Here's how the part is built. I have some questions about the finished solid (model axes, mm). A direction names the side the tool comes from. Give positions to 0.01 mm unless a question says otherwise; leave off trailing zeros. Loops run counter-clockwise (first coordinate to the right, second up) from the corner with the lowest first, then second, coordinate; pieces in that order, holes last. Notation, with made-up numbers: (44.25, 22.5) -> (61.25, 22.5) arc R34 cw to (61.25, 60.5) -> close; hole circle Ø10 at (26, 46.25). An arc over 180 degrees is marked (long way). Answer in a Markdown table with one row per item. Add a question column.
Item 1: If I drill on line 1 (X direction, y = 13, z = 66.5); line 2 (Y direction, x = -5, z = 61); line 3 (X direction, y = -24, z = 64.75), over which ranges is the centre line in solid material (lowest first)?
Item 2: If we section it at A-A (y = 0): Write out the boundary of the cut face in (x, z) (3 decimals), then the cut area to 3 significant figures.
Item 3: We'd pull the mould along Y, two halves only. Please class faces 6 (the face through (0, 13.5, 46)), 7 (the face through (0, -16, 55)), 8 (the face through (-1.172, 8.923, 53.591)), 9 (the face through (0, -13.5, 56)): released by +Y, released by -Y, zero draft, split by the parting line, or undercut.
Item 4: Which directions (+Z, -Z, +X, -X, +Y, -Y) give clear straight access to the entire face, cutting with the end or side of a thin tool? Please do faces 1 (the face through (0, 10, 65)), 2 (the face through (-14.2, 10.1, 63)), 3 (the face through (0, -13.5, 46)), 4 (the face through (0, -18.5, 51)), 5 (the face through (8.73, 6.69, 45.67)).
Item 5: If we section it at D-D (y = -6): Write out the boundary of the cut face in (x, z).
Item 6: For P1, Ø5, axis at x = 9.5, z = 47.5, coming from the -Y side; P2, Ø12, axis at x = 13, z = 58, coming from the +Y side; P3, Ø5, axis at x = -1.5, y = -3, coming from the -Z side; P4, Ø1, axis at y = 1, z = 47, coming from the +X side, each with a flat end and sliding along its axis, tell me the tip position at first contact or that it passes through.
Item 7: If we section it at C-C (y = -24): Write out the boundary of the cut face in (x, z), then the cut area to 3 significant figures.
```python
from build123d import *

# Parameters (mm, degrees)
BOSS_EXTRUDE1_DEPTH      = 13.5
BOSS_EXTRUDE2_DEPTH      = 18.5
BOSS_EXTRUDE3_DEPTH      = 5
SKETCH4_W                = 45.922011884
SKETCH4_H                = 20
BOSS_EXTRUDE4_DEPTH      = 13.5
SKETCH2_R                = 4
CUT_EXTRUDE1_DEPTH       = 268.629329099
SKETCH5_R                = 8
CUT_EXTRUDE2_DEPTH       = 4
SKETCH6_R                = 9
CUT_EXTRUDE3_DEPTH       = 12
SKETCH7_R                = 12.5
CUT_EXTRUDE4_DEPTH       = 5
BOSS_EXTRUDE5_DEPTH      = 13.5
CUT_EXTRUDE5_REACH       = 210.1
CUT_EXTRUDE5_END_RADIUS  = 45
SKETCH8_R                = 9
CUT_EXTRUDE6_REACH       = 210.1
SKETCH10_R               = 4.5
SKETCH18_R               = 11
CUT_EXTRUDE9_DEPTH       = 47
CUT_EXTRUDE10_DEPTH      = 268.629329099
CUT_EXTRUDE10_DEPTH_BACK = 268.629329099
SKETCH19_W               = 45.922011884
SKETCH19_H               = 198
SKETCH30_R               = 8.025
CUT_EXTRUDE13_DEPTH      = 4
BOSS_EXTRUDE9_DEPTH      = 16
M5_TAPPED_HOLE2_D        = 4.2
CUT_EXTRUDE17_DEPTH      = 3
M2_TAPPED_HOLE1_D        = 1.6
M2_TAPPED_HOLE1_DEPTH    = 8
M2_TAPPED_HOLE1_TIP      = 0.480688495


with BuildPart() as part:
    # Sketch1 → Boss-Extrude1 (new, symmetric)
    with BuildSketch(Plane(origin=(0, 0, 0), x_dir=(1, 0, 0), z_dir=(0, 1, 0))):
        with BuildLine():
            ThreePointArc((17.220754456, -41.574578963), (0, -45), (-17.220754456, -41.574578963))
            Line((-17.220754456, -41.574578963), (-22.961005942, -55.432771951))
            ThreePointArc((-22.961005942, -55.432771951), (0, -60), (22.961005942, -55.432771951))
            Line((22.961005942, -55.432771951), (17.220754456, -41.574578963))
        make_face()
    extrude(amount=BOSS_EXTRUDE1_DEPTH, both=True)

    # Sketch1_3 → Boss-Extrude2 (add, symmetric)
    with BuildSketch(Plane(origin=(0, 0, 0), x_dir=(1, 0, 0), z_dir=(0, 1, 0))):
        with BuildLine():
            ThreePointArc((19.134171618, -46.193976626), (0, -50), (-19.134171618, -46.193976626))
            Line((-19.134171618, -46.193976626), (-21.04758878, -50.813374288))
            ThreePointArc((-21.04758878, -50.813374288), (0, -55), (21.04758878, -50.813374288))
            Line((21.04758878, -50.813374288), (19.134171618, -46.193976626))
        make_face()
    extrude(amount=BOSS_EXTRUDE2_DEPTH, both=True)

    # Sketch3 → Boss-Extrude3 (add, symmetric)
    with BuildSketch(Plane.XZ):
        with BuildLine():
            Line((-22.961005942, 266), (-22.961005942, 55.432771951))
            ThreePointArc((-22.961005942, 55.432771951), (-20.481139434, 56.39612511), (-17.961005942, 57.248600555))
            Line((-17.961005942, 57.248600555), (-17.961005942, 246))
            Line((-17.961005942, 246), (17.961005942, 246))
            Line((17.961005942, 246), (17.961005942, 57.248600555))
            ThreePointArc((17.961005942, 57.248600555), (20.481139434, 56.39612511), (22.961005942, 55.432771951))
            Line((22.961005942, 55.432771951), (22.961005942, 266))
            Line((22.961005942, 266), (-22.961005942, 266))
        make_face()
    extrude(amount=BOSS_EXTRUDE3_DEPTH, both=True)

    # Sketch4 → Boss-Extrude4 (add, symmetric)
    with BuildSketch(Plane(origin=(0, 0, 0), x_dir=(1, 0, 0), z_dir=(0, 1, 0))):
        with Locations((0, -256)):
            Rectangle(SKETCH4_W, SKETCH4_H)
    extrude(amount=BOSS_EXTRUDE4_DEPTH, both=True)

    # Sketch2 → Cut-Extrude1 (cut, through all)
    with BuildSketch(Plane.XY):
        with Locations(Location((0, 0, 0), (0, 0, 180))):
            Circle(SKETCH2_R)
    extrude(amount=CUT_EXTRUDE1_DEPTH, mode=Mode.SUBTRACT)

    # Sketch5 → Cut-Extrude2 (cut)
    with BuildSketch(Plane(origin=(0, 0, 246), x_dir=(-1, 0, 0), z_dir=(0, 0, -1))):
        Circle(SKETCH5_R)
    extrude(amount=-CUT_EXTRUDE2_DEPTH, mode=Mode.SUBTRACT)

    # Sketch6 → Cut-Extrude3 (cut)
    with BuildSketch(Plane.XY.offset(266)):
        Circle(SKETCH6_R)
    extrude(amount=-CUT_EXTRUDE3_DEPTH, mode=Mode.SUBTRACT)

    # Sketch7 → Cut-Extrude4 (cut)
    with BuildSketch(Plane.XY.offset(266)):
        Circle(SKETCH7_R)
    extrude(amount=-CUT_EXTRUDE4_DEPTH, mode=Mode.SUBTRACT)

    # Sketch9 → Boss-Extrude5 (add, symmetric)
    with BuildSketch(Plane(origin=(0, 0, 0), x_dir=(1, 0, 0), z_dir=(0, 1, 0))):
        with BuildLine():
            Line((-22.961005942, -55.432771951), (-22.961005942, -68))
            Line((-22.961005942, -68), (22.961005942, -68))
            Line((22.961005942, -68), (22.961005942, -55.432771951))
            ThreePointArc((22.961005942, -55.432771951), (0, -60), (-22.961005942, -55.432771951))
        make_face()
    extrude(amount=BOSS_EXTRUDE5_DEPTH, both=True)

    # Cut-Extrude5: up to this cylinder (the profile starts outside it)
    cut_extrude5_end = Plane(origin=(0, 0, 0), z_dir=(0, -1, 0)) * Cylinder(CUT_EXTRUDE5_END_RADIUS, 511.2, mode=Mode.PRIVATE)
    # Sketch8 → Cut-Extrude5 (cut, up to the surface)
    with BuildSketch(Plane.XY.offset(60), mode=Mode.PRIVATE) as cut_extrude5_sk1:
        Circle(SKETCH8_R)
    cut_extrude5_tool1 = extrude(cut_extrude5_sk1.sketch, amount=-CUT_EXTRUDE5_REACH, mode=Mode.PRIVATE) - cut_extrude5_end
    add(cut_extrude5_tool1.solids().sort_by_distance((0, 0, 60))[0], mode=Mode.SUBTRACT)

    # Sketch10 → Cut-Extrude6 (cut, up to next)
    with BuildSketch(Plane.XY.offset(60), mode=Mode.PRIVATE) as cut_extrude6_sk1:
        with Locations(Location((0, 0, 0), (0, 0, 180))):
            Circle(SKETCH10_R)
    cut_extrude6_tool1 = extrude(cut_extrude6_sk1.sketch, amount=CUT_EXTRUDE6_REACH, mode=Mode.PRIVATE) & part.part
    add(cut_extrude6_tool1.solids().sort_by_distance((0, 0, 60))[0], mode=Mode.SUBTRACT)

    # Sketch18 → Cut-Extrude9 (cut)
    with BuildSketch(Plane.XY):
        with Locations(Location((0, 0, 0), (0, 0, 180))):
            Circle(SKETCH18_R)
    extrude(amount=CUT_EXTRUDE9_DEPTH, mode=Mode.SUBTRACT)

    # Sketch19 → Cut-Extrude10 (cut, two sides: drawn at the far end of the back side and taken through both)
    with BuildSketch(Plane(origin=(0, 0, 0), x_dir=(1, 0, 0), z_dir=(0, 1, 0)).offset(-CUT_EXTRUDE10_DEPTH_BACK)):
        with Locations((0, -167)):
            Rectangle(SKETCH19_W, SKETCH19_H)
    extrude(amount=CUT_EXTRUDE10_DEPTH + CUT_EXTRUDE10_DEPTH_BACK, mode=Mode.SUBTRACT)

    # Sketch23 → M5 Tapped Hole1 (revolve, cut)
    with BuildSketch(Plane(origin=(14.26606865, 8, 68), x_dir=(0, -1, 0), z_dir=(1, 0, 0))):
        Polygon((0, 0), (0, 11.3618073), (2.1, 10.1), (2.1, 0), align=None)
    m5_tapped_hole1 = revolve(axis=Axis((14.26606865, 8, 74.35), (0, 0, -1)), mode=Mode.SUBTRACT)

    # Mirror1: M5 Tapped Hole1 across plane
    add(m5_tapped_hole1.mirror(Plane(origin=(0, 0, 0), x_dir=(0, 0, 1), z_dir=(1, 0, 0))), mode=Mode.SUBTRACT)

    # Sketch30 → Cut-Extrude13 (cut)
    with BuildSketch(Plane(origin=(0, 0, 60), x_dir=(-1, 0, 0), z_dir=(0, 0, -1))):
        Circle(SKETCH30_R)
    extrude(amount=-CUT_EXTRUDE13_DEPTH, mode=Mode.SUBTRACT)

    # Sketch37 → Boss-Extrude9 (add)
    with BuildSketch(Plane.XZ.offset(13.5)):
        with BuildLine():
            Line((-22.961005942, 68), (22.961005942, 68))
            Line((22.961005942, 68), (22.961005942, 57))
            ThreePointArc((22.961005942, 57), (0, 61.450856738), (-22.961005942, 57))
            Line((-22.961005942, 57), (-22.961005942, 68))
        make_face()
    extrude(amount=BOSS_EXTRUDE9_DEPTH)

    # M5 Tapped Hole2 (through all)
    with Locations(Plane.XY.offset(68)):
        with Locations((-14.26606865, -24), (14.26606865, -24)):
            Hole(M5_TAPPED_HOLE2_D / 2)

    # Sketch40 → Cut-Extrude17 (cut)
    with BuildSketch(Plane.XY.offset(68)):
        with BuildLine():
            Line((-7, 13.5), (-7, 8))
            ThreePointArc((-7, 8), (-6.560660172, 6.939339828), (-5.5, 6.5))
            Line((-5.5, 6.5), (5.5, 6.5))
            ThreePointArc((5.5, 6.5), (6.560660172, 6.939339828), (7, 8))
            Line((7, 8), (7, 13.5))
            Line((7, 13.5), (-7, 13.5))
        make_face()
    extrude(amount=-CUT_EXTRUDE17_DEPTH, mode=Mode.SUBTRACT)

    # M2 Tapped Hole1
    with Locations(Plane.XY.offset(65)):
        with Locations((5, 10.5), (-5, 10.5)):
            Hole(M2_TAPPED_HOLE1_D / 2, depth=M2_TAPPED_HOLE1_DEPTH)
            with Locations((0, 0, -(M2_TAPPED_HOLE1_DEPTH + M2_TAPPED_HOLE1_TIP / 2))):  # 118° drill point
                Cone(0, M2_TAPPED_HOLE1_D / 2, M2_TAPPED_HOLE1_TIP, mode=Mode.SUBTRACT)


solid = part.part
```
Recorded:
| question | item | result |
|---|---|---|
| 1 | line 1 | x = -22.96 to -7, 7 to 22.96 |
| 1 | line 2 | y = -13.5 to -6.28, 6.28 to 9.7, 11.3 to 13.5 |
| 1 | line 3 | x = -22.96 to -16.37, -12.17 to 12.17, 16.37 to 22.96 |
| 2 | outline | (-22.961, 55.433) -> (-17.221, 41.575) arc R45 cw to (-11, 43.635) -> (-11, 47) -> (-9, 47) -> (-9, 60) -> (-8.025, 60) -> (-8.025, 64) -> (-4.5, 64) -> (-4.5, 68) -> (-22.961, 68) -> close; (4.5, 64) -> (8.025, 64) -> (8.025, 60) -> (9, 60) -> (9, 47) -> (11, 47) -> (11, 43.635) arc R45 cw to (17.221, 41.575) -> (22.961, 55.433) -> (22.961, 68) -> (4.5, 68) -> close |
| 2 | area | 667 mm^2 |
| 3 | face 6 | released by +Y |
| 3 | face 7 | zero draft |
| 3 | face 8 | undercut |
| 3 | face 9 | released by -Y |
| 4 | face 1 | +Z, +Y |
| 4 | face 2 | +Z |
| 4 | face 3 | -Z, -Y |
| 4 | face 4 | -Z, +X, -X, -Y |
| 4 | face 5 | -Z |
| 5 | outline | (-22.96, 55.43) -> (-17.22, 41.57) arc R45 cw to (-9.22, 44.05) -> (-9.22, 47) -> (-6.71, 47) -> (-6.71, 60) -> (-5.33, 60) -> (-5.33, 64) -> (5.33, 64) -> (5.33, 60) -> (6.71, 60) -> (6.71, 47) -> (9.22, 47) -> (9.22, 44.05) arc R45 cw to (17.22, 41.57) -> (22.96, 55.43) -> (22.96, 68) -> (-22.96, 68) -> close |
| 6 | P1 | stops at y = -18.5 |
| 6 | P2 | stops at y = 18.5 |
| 6 | P3 | stops at z = 64 |
| 6 | P4 | stops at x = 19.68 |
| 7 | outline | (-22.96, 57) arc R61.45 cw to (-16.37, 59.23) -> (-16.37, 68) -> (-22.96, 68) -> close; (-12.17, 60.23) arc R61.45 cw to (12.17, 60.23) -> (12.17, 68) -> (-12.17, 68) -> close; (16.37, 59.23) arc R61.45 cw to (22.96, 57) -> (22.96, 68) -> (16.37, 68) -> close |
| 7 | area | 299 mm^2 |
